Design review of the part built by this model. Coordinates are the model's own, in mm. A direction names the side the tool comes from. Give positions to 0.01 mm unless a question says otherwise; leave off trailing zeros. Write each loop counter-clockwise with the first axis right and the second up, starting at its lowest first coordinate (ties: lowest second). Pieces come first, ordered by that corner, then holes. Notation, with made-up numbers: (59.25, 61) -> (90.25, 61) arc R35 cw to (90.25, 99) -> close; hole circle Ø10 at (29.25, 29.5). An arc over 180 degrees is marked (long way). Put each result on its own line as item: value. Start each with the question number.
from build123d import *

# Parameters (mm, degrees)
BOSS_EXTRUDE1_DEPTH = 30.8
SKETCH2_R           = 1.5
CUT_EXTRUDE1_DEPTH  = 3


with BuildPart() as part:
    # Sketch1 → Boss-Extrude1 (new body)
    with BuildSketch(Plane.XY):
        Polygon((-9.054919228, 5.785059654), (9.054919228, 5.785059654), (10.856146045, 3.983832837), (10.856146045, 1.977204652), (9.091867013, 0.21292562), (9.091867013, -0.817284255), (9.66657341, -1.391990652), (10.13460575, -1.391990652), (10.856146045, -2.113530947), (10.856146045, -3.22536771), (10.261359727, -3.820154028), (10.666709383, -4.225503683), (15.692371673, -4.225503683), (17, -2.917875356), (17, 8.301296502), (14.320116844, 10.981179658), (-14.320116844, 10.981179658), (-17, 8.301296502), (-17, -2.917875356), (-15.692371673, -4.225503683), (-10.666709383, -4.225503683), (-10.261359727, -3.820154028), (-10.856146045, -3.22536771), (-10.856146045, -2.113530947), (-10.13460575, -1.391990652), (-9.66657341, -1.391990652), (-9.091867013, -0.817284255), (-9.091867013, 0.21292562), (-10.856146045, 1.977204652), (-10.856146045, 3.983832837), align=None)
    extrude(amount=BOSS_EXTRUDE1_DEPTH)

    # Sketch2 → Cut-Extrude1 (cut)
    with BuildSketch(Plane(origin=(0, 10.981179658, 0), x_dir=(1, 0, 0), z_dir=(0, 1, 0))):
        with Locations(Location((-6, -8.9, 0), (0, 0, 270))):
            Circle(SKETCH2_R)
        with Locations(Location((6, -8.9, 0), (0, 0, 90))):
            Circle(SKETCH2_R)
        with Locations(Location((6, -21.9, 0), (0, 0, 270))):
            Circle(SKETCH2_R)
        with Locations(Location((-6, -21.9, 0), (0, 0, 90))):
            Circle(SKETCH2_R)
    extrude(amount=-CUT_EXTRUDE1_DEPTH, mode=Mode.SUBTRACT)


solid = part.part
Q1. Take a section at A-A on y = 5.25. Give the boundary of the cut face in (x, z), then the cut area to 3 significant figures.
Q2. For pin 1 (3.5 mm diameter, centred on x = -6, z = 8.9, fed in from -Y); pin 2 (2.5 mm diameter, centred on x = -5.5, z = 21.5, fed in from +Y); pin 3 (1.5 mm diameter, centred on x = -5.5, z = 9, fed in from +Y), all flat-tipped, find the tip position at first contact; note any pin that passes through.
Q3. Mouldability with a two-part tool opening along X and no side actions: class faces 6 (the face through (0, 7, 30.8)), 7 (the face through (10.856, -3, 15)), 8 (the face through (16.34, -3.58, 15.18)) as +X half, -X half, draft (parallel to the pull), parting line (faces both ways), or undercut.
Q4. Take a section at B-B on x = 6. Give the boundary of the cut face in (y, z), then the cut area to 3 significant figures.
Q5. Machinability: for faces 1 (the face through (6, 7.981, 9)), 2 (the face through (15.7, 9.6, 15.2)), 3 (the face through (13, -4.226, 15)), 4 (the face through (-9.092, 0, 15)), 5 (the face through (-10.856, -3, 15)), which of the approach directions +Z, -Z, +X, -X, +Y, -Y give a long, thin tool a straight path to every point of the face, cutting with its end or side? Answer none if there is none.
Q6. Take a section at D-D on y = 1. Give the boundary of the cut face in (x, z), then the cut area to 3 significant figures.
Q7. To check wall thickness, follow probe 1 along X at (y, z) = (10.1, 21.9); probe 2 along X at (y, z) = (10, 9); probe 3 along Y at (x, z) = (9, 18). State the ranges of each line that lie inside material, in increasing order. Write a range as from..to.
Result:
1. outline: (-17, 0) -> (-9.59, 0) -> (-9.59, 30.8) -> (-17, 30.8) -> close; (9.59, 0) -> (17, 0) -> (17, 30.8) -> (9.59, 30.8) -> close
1. area: 456 mm^2
2. pin 1: stops at y = 5.79
2. pin 2: stops at y = 10.98
2. pin 3: stops at y = 7.98
3. face 6: draft
3. face 7: undercut
3. face 8: +X half
4. outline: (5.79, 0) -> (10.98, 0) -> (10.98, 7.4) -> (7.98, 7.4) -> (7.98, 10.4) -> (10.98, 10.4) -> (10.98, 20.4) -> (7.98, 20.4) -> (7.98, 23.4) -> (10.98, 23.4) -> (10.98, 30.8) -> (5.79, 30.8) -> close
4. area: 142 mm^2
5. face 1: +Y
5. face 2: +Z, -Z, +X, +Y
5. face 3: +Z, -Z, +X, -X, -Y
5. face 4: +Z, -Z, -Y
5. face 5: +Z, -Z
6. outline: (-17, 0) -> (-9.88, 0) -> (-9.88, 30.8) -> (-17, 30.8) -> close; (9.88, 0) -> (17, 0) -> (17, 30.8) -> (9.88, 30.8) -> close
6. area: 439 mm^2
7. probe 1: x = -15.2..-7.5, -4.5..4.5, 7.5..15.2
7. probe 2: x = -15.3..-7.5, -4.5..4.5, 7.5..15.3
7. probe 3: y = 5.79..10.98
